Here's how the part is built. I have some questions about the finished solid (model axes, mm). A direction names the side the tool comes from. Coordinates: 2 decimals unless noted, no trailing zeros. Loops run counter-clockwise (first coordinate to the right, second up) from the corner with the lowest first, then second, coordinate; pieces in that order, holes last. Notation, with made-up numbers: M -18.5,67.5 L 23.5,67.5 A26 ccw 23.5,93.5 Z; hole C 52.5,56 d4. An arc over 180 degrees is marked long. Use CSV: the item, a comma, the result in double quotes. Start each with the question number.
Q1. Which directions (+Z, -Z, +X, -X, +Y, -Y) give clear straight access to the entire face, cutting with the end or side of a thin tool? Please do faces 5 (the flat face through (0, 0, 0.92)), 6 (the flat face through (0, -2, 2.3)).
Q2. If we section it at B-B (z = -4.25): Please give me the cut outline in (x, y).
Q3. For pin 1 Ø3 at (x, y) = (-3, 2) entering from -Z; pin 2 Ø1 at (x, y) = (3, -2) entering from -Z; pin 3 Ø1.5 at (x, z) = (1.5, -12.5) entering from +Y, each with a flat end and sliding along its axis, tell me the tip position at first contact or that it passes through.
Q4. If we section it at A-A (y = 0): Please give me the cut outline in (x, z) (3 decimals), and give its area (3 significant figures).
Q5. Please list where these lines run through material, in increasing order: probe 1 along Z at (x, y) = (0.75, -0.5); probe 2 along Z at (x, y) = (0.5, 2.25); probe 3 along Y at (x, z) = (2.25, 0.75). Write a range as [from, to].
Q6. If we mould it in two halves opening along Y, with no side actions, what happens to faces 1 (the cylindrical face through (2, 0, -11)), 2 (the flat face through (-0.616, 1.088, 1.62)), 3 (the flat face through (0, 0, -22.7)), 4 (the flat face through (0.616, -1.088, 1.62))? For each: +Y half, -Y half, draft (parallel to the pull), parting line (faces both ways), or undercut.
from build123d import *

# Parameters (mm, degrees)
CUT_EXTRUDE2_DEPTH = 1.38
SKETCH6_R          = 1.443375673
CUT_EXTRUDE3_DEPTH = 1.38
CUT_EXTRUDE3_TAPER = 45


with BuildPart() as part:
    # Sketch14 → Revolve1 (revolve)
    with BuildSketch(Plane(origin=(0, 0, 0), x_dir=(0, 0, -1), z_dir=(1, 0, 0))):
        Polygon((-2.3, 0), (-2.3, 4), (-2.15, 4), (-0.15, 2), (0, 2), (22.175, 2), (22.7, 1.475), (22.7, 0), align=None)
    revolve(axis=Axis((0, 0, -22.7), (0, 0, 1)))

    # Sketch5 → Cut-Extrude2 (cut)
    with BuildSketch(Plane.XY.offset(2.3)):
        Polygon((0, -1.443375673), (1.25, -0.721687836), (1.25, 0.721687836), (0, 1.443375673), (-1.25, 0.721687836), (-1.25, -0.721687836), align=None)
    extrude(amount=-CUT_EXTRUDE2_DEPTH, mode=Mode.SUBTRACT)

    # Sketch6 → Cut-Extrude3 (cut)
    with BuildSketch(Plane.XY.offset(2.3)):
        Circle(SKETCH6_R)
    extrude(amount=-CUT_EXTRUDE3_DEPTH, taper=CUT_EXTRUDE3_TAPER, mode=Mode.SUBTRACT)


solid = part.part
Results below:
1,face 5,"+Z"
1,face 6,"+Z, +X, -X, +Y, -Y"
2,outline,"C 0,0 d4"
3,pin 1,"z = 0.26"
3,pin 2,"z = 1.26"
3,pin 3,"y = 1.85"
4,outline,"M -4,2.15 L -2,0.15 L -2,-22.175 L -1.475,-22.7 L 1.475,-22.7 L 2,-22.175 L 2,0.15 L 4,2.15 L 4,2.3 L 1.443,2.3 L 1.25,2.107 L 1.25,0.92 L -1.25,0.92 L -1.25,2.107 L -1.443,2.3 L -4,2.3 Z"
4,area,"101 mm^2"
5,probe 1,"[-22.7, 0.92]"
5,probe 2,"[0.45, 2.3]"
5,probe 3,"[-1.3, 1.3]"
6,face 1,"parting line"
6,face 2,"undercut"
6,face 3,"draft"
6,face 4,"undercut"
